Geometry check sheet. Reference: drawing and pictorial views, mm from the part's lowest x, y, z. Round coordinates to 2 decimals unless told otherwise and drop trailing zeros. Write each loop counter-clockwise with the first axis right and the second up, starting at its lowest first coordinate (ties: lowest second). Pieces come first, ordered by that corner, then holes. Notation, with made-up numbers: (4.25, 23) - (20.25, 23) arc R25 cw to (20.25, 62) - close; hole circle Ø10 at (13, 48.5). An arc over 180 degrees is marked (long way). Use one line per item in the form item = value. Start each with the question number.
1) Scan lines: probe 1 along Z at (x, y) = (151.8, 0.45); probe 2 along X at (y, z) = (1.2, 50); probe 3 along X at (y, z) = (1.65, 39). Record each from-to range of solid material in increasing order.
2) Section check A-A (x = 151.8). Record the boundary of the cut face in (y, z).
3) Section check B-B (z = 50). Record the boundary of the cut face in (x, y), then the cut area to 3 significant figures.
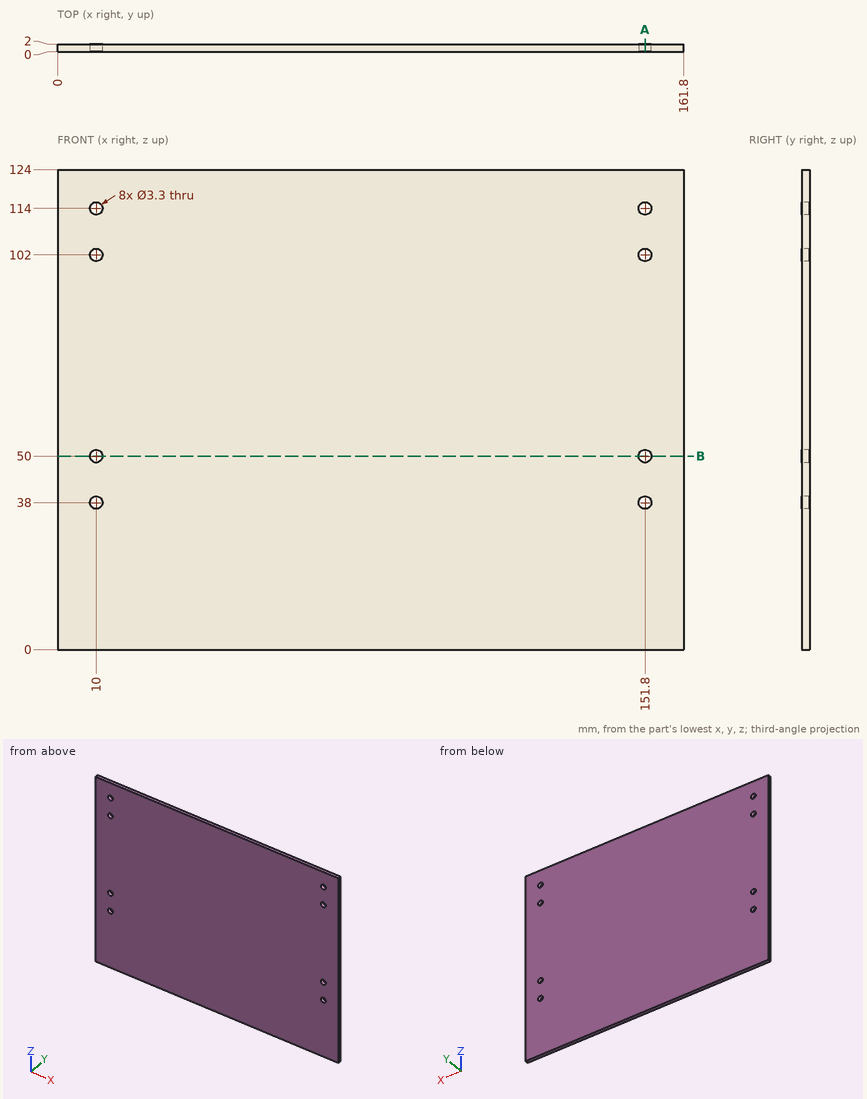
Results are:
q1.probe_1 = 0 to 36.35, 39.65 to 48.35, 51.65 to 100.35, 103.65 to 112.35, 115.65 to 124
q1.probe_2 = 0 to 8.35, 11.65 to 150.15, 153.45 to 161.8
q1.probe_3 = 0 to 8.69, 11.31 to 150.49, 153.11 to 161.8
q2.outline = (0, 0) - (2, 0) - (2, 36.35) - (0, 36.35) - close; (0, 39.65) - (2, 39.65) - (2, 48.35) - (0, 48.35) - close; (0, 51.65) - (2, 51.65) - (2, 100.35) - (0, 100.35) - close; (0, 103.65) - (2, 103.65) - (2, 112.35) - (0, 112.35) - close; (0, 115.65) - (2, 115.65) - (2, 124) - (0, 124) - close
q3.outline = (0, 0) - (8.35, 0) - (8.35, 2) - (0, 2) - close; (11.65, 0) - (150.15, 0) - (150.15, 2) - (11.65, 2) - close; (153.45, 0) - (161.8, 0) - (161.8, 2) - (153.45, 2) - close
q3.area = 310 mm²
